Part model, mm, in its own coordinate system. A direction names the side the tool comes from. Coordinates: 2 decimals unless noted, no trailing zeros. Loops run counter-clockwise (first coordinate to the right, second up) from the corner with the lowest first, then second, coordinate; pieces in that order, holes last. Notation, with made-up numbers: (-31.75, 0.25) - (8.25, 0.25) arc R36 cw to (8.25, 34.25) - close; hole circle Ø1 at (28, 54). An arc over 180 degrees is marked (long way). Use a Markdown table: item, result. Add a question column.
1) Pull direction Z, two halves, no side cores. Call faces 1 (the face through (0.5, 13.39, -1.29)), 2 (the face through (12.826, 13, 14)), 3 (the face through (0.759, 13.717, 23.048)): +Z half, -Z half, draft (parallel to the pull), parting line (faces both ways), or undercut.
2) Band-saw the part on B-B (x = 0). Give the cut face in (y, z).
3) Tool access for faces 4 (the face through (1, 12.196, 20)), 5 (the face through (0, -5.804, -1)): list every direction of +Z, -Z, +X, -X, +Y, -Y with a clear straight run to the whole face (end or side of a thin tool).
4) Band-saw the part on A-A (z = 25). Give the cut face in (x, y), plus the area to 3 significant figures.
5) Drop flat-ended pins along their axis: P1, Ø5, axis at x = -3, y = 10, coming from the -Z side; P2, Ø10, axis at x = -4, z = 31.5, coming from the -Y side; P3, Ø7.5, axis at x = 0, y = 0, coming from the +Z side; P4, Ø8, axis at x = 4, y = 6.5, coming from the +Z side. Give the stop position or say it passes through.
6) Band-saw the part on D-D (y = 6.5). Give the cut face in (x, z).
7) Band-saw the part on C-C (x = 7). Give the cut face in (y, z), plus the area to 3 significant figures.
8) Probe probe 1 along Z at (x, y) = (10, -2.75); probe 2 along Y at (x, z) = (0, -0.65); probe 3 along Y at (x, z) = (-7.75, 5). List the from-to ranges inside material, lowest first. Write a range as [from, to].
from build123d import *

# Parameters (mm, degrees)
SKETCH1_W                 = 25
SKETCH1_H                 = 15
SKETCH1_R                 = 2
BASE_FLANGE1_DEPTH        = 3
EDGE_FLANGE1_DEPTH        = 25
EDGE_FLANGE1_START        = 3
EDGE_FLANGE1_PROFILE_W    = 25
EDGE_FLANGE1_PROFILE_H    = 34
EDGE_FLANGE1_PROFILE_R    = 2
EDGE_FLANGE1_FLAT_DEPTH   = 3
BREAK_CORNER1_START       = -12.712257412
BREAK_CORNER1_OUTLINE_W   = 19.637623744
BREAK_CORNER1_OUTLINE_H   = 3
BREAK_CORNER1_DEPTH       = 3.535533905
BREAK_CORNER1_START_2     = 1.429878211
BREAK_CORNER1_2_OUTLINE_W = 4.362376256
BREAK_CORNER1_2_OUTLINE_H = 3
BREAK_CORNER1_2_DEPTH     = 7.071067812


# Read off the part's stored shape, not the designer's step: Break-Corner1
# Sheet-metal steps are written as plain solids
with BuildPart() as part:
    # Sketch1 → Base-Flange1 (new body)
    with BuildSketch(Plane.XY):
        with Locations((0.325905683, 1.696247476)):
            Rectangle(SKETCH1_W, SKETCH1_H)
        with Locations((0, -0.803752524)):
            Circle(SKETCH1_R, mode=Mode.SUBTRACT)
    extrude(amount=-BASE_FLANGE1_DEPTH)

    # Edge-Flange1 bend section (across the edge) → Edge-Flange1 (add)
    with BuildSketch(Plane(origin=(12.825905683, 12.196247476, 0), x_dir=(0, -1, 0), z_dir=(-1, 0, 0))):
        with BuildLine():
            Line((-3, 3), (0, 3))
            ThreePointArc((0, 3), (0.878679656, 0.878679656), (3, 0))
            Line((3, 0), (3, -3))
            ThreePointArc((3, -3), (-1.242640687, -1.242640687), (-3, 3))
        make_face()
    extrude(amount=EDGE_FLANGE1_DEPTH)

    # Edge-Flange1 profile (on flange) → Edge-Flange1 flat (add)
    with BuildSketch(Plane(origin=(0, 12.196247476, 0), x_dir=(-1, 0, 0), z_dir=(0, 1, 0)).offset(EDGE_FLANGE1_START)):
        with Locations((-0.325905683, 20)):
            Rectangle(EDGE_FLANGE1_PROFILE_W, EDGE_FLANGE1_PROFILE_H)
        with Locations((-0.325905683, 25)):
            Circle(EDGE_FLANGE1_PROFILE_R, mode=Mode.SUBTRACT)
    extrude(amount=-EDGE_FLANGE1_FLAT_DEPTH)

    # Break-Corner1 outline → Break-Corner1 (cut)
    with BuildSketch(Plane(origin=(0, 0, 0), x_dir=(0.707106781186548, -0.707106781186547, 0), z_dir=(0.707106781186547, 0.707106781186548, 0)).offset(BREAK_CORNER1_START)):
        with Locations((-0.181188128, 1.5)):
            Rectangle(BREAK_CORNER1_OUTLINE_W, BREAK_CORNER1_OUTLINE_H)
    extrude(amount=BREAK_CORNER1_DEPTH, mode=Mode.SUBTRACT)

    # Break-Corner1 2 outline → Break-Corner1 2 (cut)
    with BuildSketch(Plane(origin=(0, 0, 0), x_dir=(0.707106781186548, -0.707106781186547, 0), z_dir=(0.707106781186547, 0.707106781186548, 0)).offset(BREAK_CORNER1_START_2)):
        with Locations((11.818811872, 1.5)):
            Rectangle(BREAK_CORNER1_2_OUTLINE_W, BREAK_CORNER1_2_OUTLINE_H)
    extrude(amount=BREAK_CORNER1_2_DEPTH, mode=Mode.SUBTRACT)


solid = part.part
Answer block:
| question | item | result |
|---|---|---|
| 1 | face 1 | -Z half |
| 1 | face 2 | draft |
| 1 | face 3 | undercut |
| 2 | outline | (-5.8, -3) - (-2.8, -3) - (-2.8, 0) - (-5.8, 0) - close; (1.2, -3) - (9.2, -3) arc R6 ccw to (15.2, 3) - (15.2, 23.03) - (12.2, 23.03) - (12.2, 3) arc R3 cw to (9.2, 0) - (1.2, 0) - close; (12.2, 26.97) - (15.2, 26.97) - (15.2, 37) - (12.2, 37) - close |
| 3 | face 4 | +Z, +X, -X, -Y |
| 3 | face 5 | +Z, -Z, +X, -X, -Y |
| 4 | outline | (-12.17, 12.2) - (-1.67, 12.2) - (-1.67, 15.2) - (-12.17, 15.2) - close; (2.33, 12.2) - (12.83, 12.2) - (12.83, 15.2) - (2.33, 15.2) - close |
| 4 | area | 63.0 mm2 |
| 5 | P1 | z = -3 |
| 5 | P2 | y = 12.2 |
| 5 | P3 | z = 0 |
| 5 | P4 | z = 0.3 |
| 6 | outline | (-12.17, -3) - (12.83, -3) - (12.83, 0) - (-12.17, 0) - close |
| 7 | outline | (-5.8, -3) - (9.2, -3) arc R6 ccw to (15.2, 3) - (15.2, 37) - (12.2, 37) - (12.2, 3) arc R3 cw to (9.2, 0) - (-5.8, 0) - close |
| 7 | area | 168 mm2 |
| 8 | probe 1 | [-3, 0] |
| 8 | probe 2 | [-5.8, -2.8], [1.2, 13.96] |
| 8 | probe 3 | [12.2, 15.2] |
